Part print with two shaded views. Sizes in mm from the minimum x, y, z corner. A direction names the side the tool comes from. Round coordinates to 2 decimals unless told otherwise and drop trailing zeros. Order: outer loops, then holes, each group sorted by start corner. A loop starts at its lowest first (then second) coordinate and runs counter-clockwise, first axis right, second up. Notation, with made-up numbers: (37, -15.5) - (63, -15.5) arc R18 cw to (63, 4.5) - close; hole circle Ø11 at (-13, 38). An arc over 180 degrees is marked (long way). Use one line per item in the form item = value.
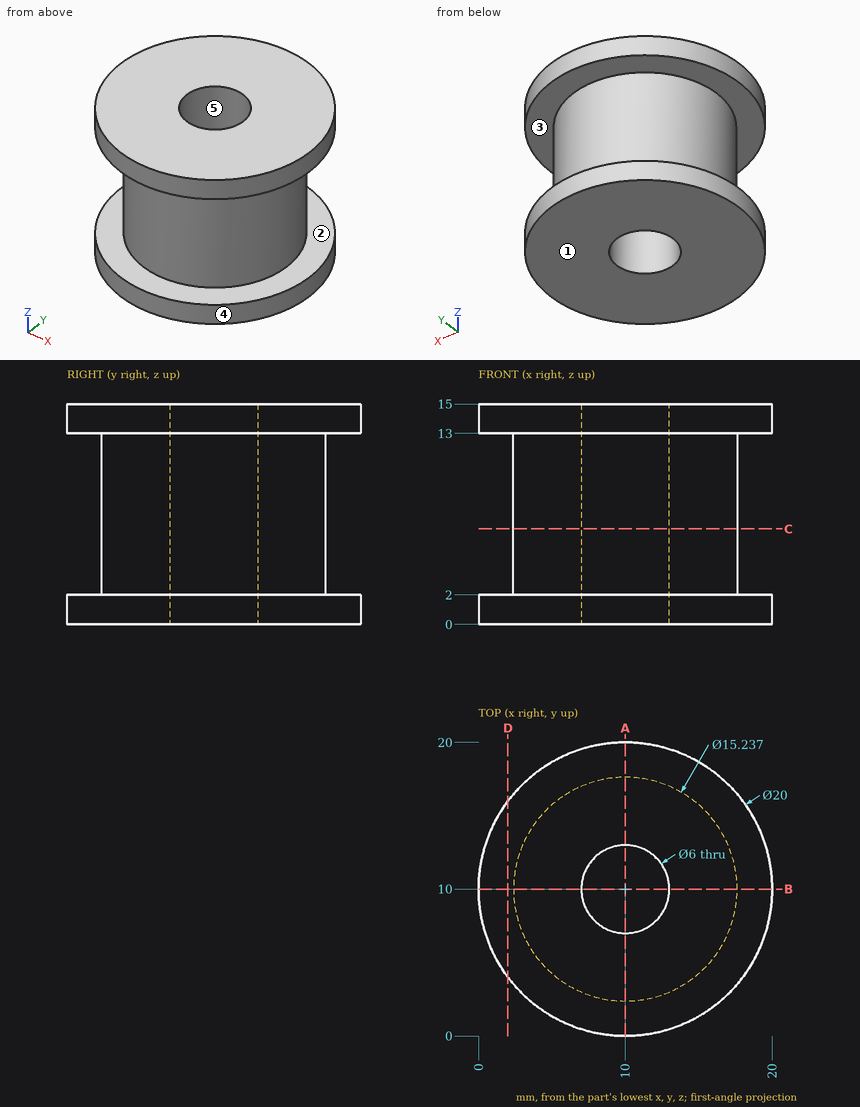
(1) Slice it at C-C on z = 6.5. Give the cut face in (x, y).
Report:
outline = circle Ø15.24 at (10, 10); hole circle Ø6 at (10, 10)
(2) Slice it at D-D on x = 2. Give the cut face in (y, z), then the cut area to 3 significant figures.
Report:
outline = (4, 0) - (16, 0) - (16, 2) - (4, 2) - close; (4, 13) - (16, 13) - (16, 15) - (4, 15) - close
area = 48.0 mm2
(3) Tool access for the marked faces 1 and 2: list every direction of +Z, -Z, +X, -X, +Y, -Y with a clear straight run to the whole face (end or side of a thin tool).
Report:
face_1 = -Z, +X, -X, +Y, -Y
face_2 = none
(4) Slice it at A-A on x = 10. Give the cut face in (y, z).
Report:
outline = (0, 0) - (7, 0) - (7, 15) - (0, 15) - (0, 13) - (2.38, 13) - (2.38, 2) - (0, 2) - close; (13, 0) - (20, 0) - (20, 2) - (17.62, 2) - (17.62, 13) - (20, 13) - (20, 15) - (13, 15) - close
(5) Pull direction X, two halves, no side cores. Call the marked faces 3, 4 and 5: released by +X, released by -X, zero draft, split by the parting line, or undercut.
Report:
face_3 = zero draft
face_4 = split by the parting line
face_5 = undercut
(6) Probe probe 1 along Z at (x, y) = (18, 6.5); probe 2 along Y at (x, z) = (10, 4); probe 3 along Y at (x, z) = (8, 11.25). List the from-to ranges inside material, lowest first. Write a range as [from, to].
Report:
probe_1 = [0, 2], [13, 15]
probe_2 = [2.38, 7], [13, 17.62]
probe_3 = [2.65, 7.76], [12.24, 17.35]
(7) Pin check, flat tip, straight feed: pin 1 (1.5 mm diameter, centred on y = 7, z = 5, fed in from +X). Stop position of the tip, or through.
Report:
pin_1 = 17.28
